Read the model definition and answer for the solid it produces. Units are mm, in the model's axes. Face numbers are marked on the shaded views. Coordinates: 2 decimals unless noted, no trailing zeros. Loops run counter-clockwise (first coordinate to the right, second up) from the corner with the lowest first, then second, coordinate; pieces in that order, holes last. Notation, with made-up numbers: (-35, 2) -> (-1, 2) arc R17 ccw to (-1, 35) -> close; hole circle Ø11 at (65, -11). An arc over 180 degrees is marked (long way). Answer as a JSON object with one key per item and string values. Group by question number.
Q1. Determine the mould class of the marked faces 1, 2, 3 and 4 for opening direction Y: released by +Y, released by -Y, zero draft, split by the parting line, or undercut.
Q2. Straight lines are drawn through the part: line 1 along Y through (x, z) = (0, -3.3) (3 decimals); line 2 along Z through (x, y) = (0, 10.5) (3 decimals); line 3 along Y through (x, z) = (3, -7). For each, find the intervals that lie inside material, in ascending order. Write a range as [from, to].
Q3. The part is cut by section D-D on x = 0.75. Write down the section's boundary in (y, z).
Q4. The part is cut by section B-B on y = 10.25. Write down the section's boundary in (x, z) (3 decimals), and give its area (3 significant figures).
Q5. The part is cut by section A-A on y = 7. Write down the section's boundary in (x, z) (3 decimals).
Q6. Each of these flat-tipped pins is pushed along its axis until it touches: P1, Ø2.5, axis at x = 0, y = 10, coming from the -Z side; P2, Ø6, axis at y = 9.5, z = 12.5, coming from the -X side; P3, Ø4, axis at x = 1.5, z = 11, coming from the -Y side. Where does it stop, or does it pass through?
Q7. The part is cut by section C-C on z = -4. Write down the section's boundary in (x, y) (3 decimals), and give its area (3 significant figures).
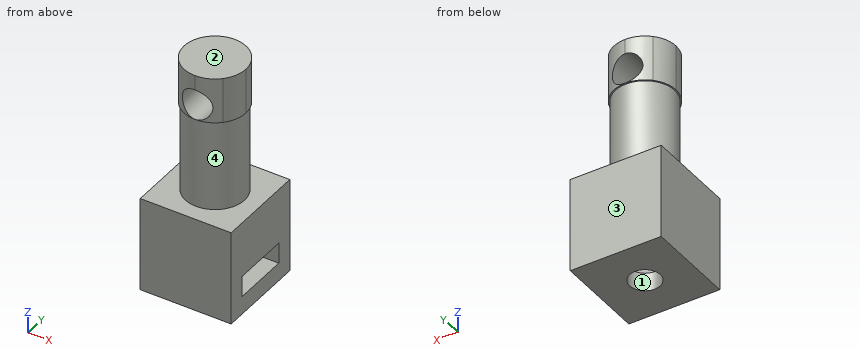
from build123d import *

# Parameters (mm, degrees)
SKETCH1_W               = 10
SKETCH1_H               = 10
BOSS_EXTRUDE1_DEPTH     = 5
CUT_EXTRUDE1_DEPTH      = 9.660254038
CUT_EXTRUDE1_DEPTH_BACK = 9.660254038
SKETCH2_R               = 1.675
SKETCH3_R               = 1.675
CUT_EXTRUDE3_DEPTH      = 2.3
SKETCH4_W               = 10
SKETCH4_H               = 10
BOSS_EXTRUDE2_DEPTH     = 2.7
SKETCH6_W               = 10
SKETCH6_H               = 10
BOSS_EXTRUDE3_DEPTH     = 7
SKETCH9_R               = 2.15
CUT_EXTRUDE12_DEPTH     = 19.468622038
SKETCH10_R              = 1.675
CUT_EXTRUDE13_DEPTH     = 13.003749414
BOSS_EXTRUDE4_DEPTH     = 2.3
SKETCH12_W              = 10
SKETCH12_H              = 10
BOSS_EXTRUDE5_DEPTH     = 2.7
CUT_EXTRUDE14_START     = -2.7
SKETCH13_R              = 1.675
CUT_EXTRUDE14_DEPTH     = 2.7
SKETCH14_R              = 2.15
BOSS_EXTRUDE6_DEPTH     = 0.76
SKETCH16_W              = 10
SKETCH16_H              = 19.7
CUT_EXTRUDE15_DEPTH     = 2.29
BOSS_EXTRUDE7_START     = 1
SKETCH17_W              = 10
SKETCH17_H              = 7.71
SKETCH17_R              = 1.675
BOSS_EXTRUDE7_DEPTH     = 1
SKETCH18_W              = 10
SKETCH18_H              = 7.71
SKETCH18_R              = 1.675
BOSS_EXTRUDE9_DEPTH     = 1
BOSS_EXTRUDE13_DEPTH    = 2.3
SKETCH23_W              = 10
SKETCH23_H              = 10
SKETCH23_R              = 1.675
BOSS_EXTRUDE15_DEPTH    = 2
SKETCH24_W              = 10
SKETCH24_H              = 5.85
CUT_EXTRUDE16_DEPTH     = 25.448519432
SKETCH25_W              = 10
SKETCH25_H              = 10
BOSS_EXTRUDE16_DEPTH    = 6
SKETCH26_W              = 10
SKETCH26_H              = 10
CUT_EXTRUDE17_DEPTH     = 7.71
SKETCH27_W              = 10
SKETCH27_H              = 10
BOSS_EXTRUDE17_DEPTH    = 6.1
SKETCH28_R              = 3.25
BOSS_EXTRUDE18_DEPTH    = 10
SKETCH29_R              = 1.625
CUT_EXTRUDE18_DEPTH     = 2.7
SKETCH33_W              = 6.8
SKETCH33_H              = 6.8
BOSS_EXTRUDE19_DEPTH    = 5
SKETCH36_R              = 1.675
CUT_EXTRUDE22_DEPTH     = 10
CUT_EXTRUDE23_DEPTH     = 10


with BuildPart() as part:
    # Sketch1 → Boss-Extrude1 (new body)
    with BuildSketch(Plane(origin=(0, 0, 0), x_dir=(1, 0, 0), z_dir=(0, 1, 0))):
        Rectangle(SKETCH1_W, SKETCH1_H)
    extrude(amount=BOSS_EXTRUDE1_DEPTH)

    # Sketch2 → Cut-Extrude1 (cut, two sides: drawn at the far end of the back side and taken through both)
    with BuildSketch(Plane(origin=(0, 5, 0), x_dir=(1, 0, 0), z_dir=(0, 1, 0)).offset(-CUT_EXTRUDE1_DEPTH_BACK)):
        with Locations(Location((0, 0, 0), (0, 0, 270))):
            Circle(SKETCH2_R)
    extrude(amount=CUT_EXTRUDE1_DEPTH + CUT_EXTRUDE1_DEPTH_BACK, mode=Mode.SUBTRACT)

    # Sketch3 → Cut-Extrude3 (cut)
    # profile 1 of 2: a face of its own
    with BuildSketch(Plane(origin=(0, 5, 0), x_dir=(1, 0, 0), z_dir=(0, 1, 0))):
        Polygon((-1.56461923, -2.71), (1.56461923, -2.71), (3.129238459, 0), (1.56461923, 2.71), (-1.56461923, 2.71), (-3.129238459, 0), align=None)
        with Locations(Location((0, 0, 0), (0, 0, 270))):
            Circle(SKETCH3_R, mode=Mode.SUBTRACT)
    # profile 2 of 2: a face of its own
    with BuildSketch(Plane(origin=(0, 5, 0), x_dir=(1, 0, 0), z_dir=(0, 1, 0))):
        Polygon((-1.56461923, -2.71), (-3.129238459, 0), (-3.129238459, -5), (3.129238459, -5), (3.129238459, 0), (1.56461923, -2.71), align=None)
    extrude(amount=-CUT_EXTRUDE3_DEPTH, mode=Mode.SUBTRACT)

    # Sketch4 → Boss-Extrude2 (add)
    with BuildSketch(Plane(origin=(0, 5, 0), x_dir=(1, 0, 0), z_dir=(0, 1, 0))):
        Rectangle(SKETCH4_W, SKETCH4_H)
    extrude(amount=BOSS_EXTRUDE2_DEPTH)

    # Sketch6 → Boss-Extrude3 (add)
    with BuildSketch(Plane(origin=(0, 7.7, 0), x_dir=(1, 0, 0), z_dir=(0, 1, 0))):
        Rectangle(SKETCH6_W, SKETCH6_H)
    extrude(amount=BOSS_EXTRUDE3_DEPTH)

    # Sketch9 → Cut-Extrude12 (cut, through all)
    with BuildSketch(Plane(origin=(0, 0, -5), x_dir=(-1, 0, 0), z_dir=(0, 0, -1))):
        with Locations((0, 9.85)):
            Circle(SKETCH9_R)
    extrude(amount=-CUT_EXTRUDE12_DEPTH, mode=Mode.SUBTRACT)

    # Sketch10 → Cut-Extrude13 (cut, through all)
    with BuildSketch(Plane.XZ.offset(-5)):
        with Locations(Location((0, 0, 0), (0, 0, 90))):
            Circle(SKETCH10_R)
    extrude(amount=-CUT_EXTRUDE13_DEPTH, mode=Mode.SUBTRACT)

    # Sketch11 → Boss-Extrude4 (add)
    with BuildSketch(Plane(origin=(0, 14.7, 0), x_dir=(1, 0, 0), z_dir=(0, 1, 0))):
        Polygon((1.56461923, 2.71), (3.129238459, 0), (3.129238459, -5), (5, -5), (5, 5), (-5, 5), (-5, -5), (-3.129238459, -5), (-3.129238459, 0), (-1.56461923, 2.71), align=None)
    extrude(amount=BOSS_EXTRUDE4_DEPTH)

    # Sketch12 → Boss-Extrude5 (add)
    with BuildSketch(Plane(origin=(0, 17, 0), x_dir=(1, 0, 0), z_dir=(0, 1, 0))):
        Rectangle(SKETCH12_W, SKETCH12_H)
    extrude(amount=BOSS_EXTRUDE5_DEPTH)

    # Sketch13 → Cut-Extrude14 (cut)
    with BuildSketch(Plane(origin=(0, 19.7, 0), x_dir=(1, 0, 0), z_dir=(0, 1, 0)).offset(CUT_EXTRUDE14_START)):
        with Locations(Location((0, 0, 0), (0, 0, 270))):
            Circle(SKETCH13_R)
    extrude(amount=CUT_EXTRUDE14_DEPTH, mode=Mode.SUBTRACT)

    # Sketch16 → Cut-Extrude15 (cut)
    with BuildSketch(Plane.XY.offset(5)):
        with Locations((0, 9.85)):
            Rectangle(SKETCH16_W, SKETCH16_H)
    extrude(amount=-CUT_EXTRUDE15_DEPTH, mode=Mode.SUBTRACT)

    # Sketch17 → Boss-Extrude7 (add)
    with BuildSketch(Plane(origin=(0, 0, 0), x_dir=(-1, 0, 0), z_dir=(0, -1, 0)).offset(BOSS_EXTRUDE7_START)):
        with Locations((0, 1.145)):
            Rectangle(SKETCH17_W, SKETCH17_H)
        with Locations(Location((0, 0, 0), (0, 0, 270))):
            Circle(SKETCH17_R, mode=Mode.SUBTRACT)
    extrude(amount=-BOSS_EXTRUDE7_DEPTH)

    # Sketch18 → Boss-Extrude9 (add)
    with BuildSketch(Plane(origin=(0, 19.7, 0), x_dir=(1, 0, 0), z_dir=(0, 1, 0))):
        with Locations((0, 1.145)):
            Rectangle(SKETCH18_W, SKETCH18_H)
        with Locations(Location((0, 0, 0), (0, 0, 270))):
            Circle(SKETCH18_R, mode=Mode.SUBTRACT)
    extrude(amount=BOSS_EXTRUDE9_DEPTH)


with BuildPart() as body_2:
    # Sketch14 → Boss-Extrude6 (new body)
    with BuildSketch(Plane(origin=(0, 0, -5), x_dir=(-1, 0, 0), z_dir=(0, 0, -1))):
        with Locations((0, 9.85)):
            Circle(SKETCH14_R)
    extrude(amount=-BOSS_EXTRUDE6_DEPTH)


    add(part.part)  # Boss-Extrude13 merges part
    # Sketch22 → Boss-Extrude13 (add)
    with BuildSketch(Plane(origin=(0, 0, -5), x_dir=(-1, 0, 0), z_dir=(0, 0, -1))):
        Polygon((-5, 12.979238459), (0, 12.979238459), (2.71, 11.41461923), (2.71, 8.28538077), (0, 6.720761541), (-5, 6.720761541), (-5, 4.85), (5, 4.85), (5, 14.85), (-5, 14.85), align=None)
    extrude(amount=BOSS_EXTRUDE13_DEPTH)

    # Sketch23 → Boss-Extrude15 (add)
    with BuildSketch(Plane(origin=(0, 0, -7.3), x_dir=(-1, 0, 0), z_dir=(0, 0, -1))):
        with Locations((0, 9.85)):
            Rectangle(SKETCH23_W, SKETCH23_H)
        with Locations((0, 9.85)):
            Circle(SKETCH23_R, mode=Mode.SUBTRACT)
    extrude(amount=BOSS_EXTRUDE15_DEPTH)

    # Sketch24 → Cut-Extrude16 (cut, through all)
    with BuildSketch(Plane(origin=(0, 0, -9.3), x_dir=(-1, 0, 0), z_dir=(0, 0, -1))):
        with Locations((0, 17.775)):
            Rectangle(SKETCH24_W, SKETCH24_H)
        with Locations((0, 1.925)):
            Rectangle(SKETCH24_W, SKETCH24_H)
    extrude(amount=-CUT_EXTRUDE16_DEPTH, mode=Mode.SUBTRACT)

    # Sketch25 → Boss-Extrude16 (add)
    with BuildSketch(Plane.XY.offset(2.71)):
        with Locations((0, 9.85)):
            Rectangle(SKETCH25_W, SKETCH25_H)
    extrude(amount=-BOSS_EXTRUDE16_DEPTH)

    # Sketch26 → Cut-Extrude17 (cut)
    with BuildSketch(Plane.XY.offset(2.71)):
        with Locations((0, 9.85)):
            Rectangle(SKETCH26_W, SKETCH26_H)
    extrude(amount=-CUT_EXTRUDE17_DEPTH, mode=Mode.SUBTRACT)

    # Sketch27 → Boss-Extrude17 (add)
    with BuildSketch(Plane.XY.offset(-5)):
        with Locations((0, 9.85)):
            Rectangle(SKETCH27_W, SKETCH27_H)
    extrude(amount=BOSS_EXTRUDE17_DEPTH)

    # Sketch28 → Boss-Extrude18 (add)
    with BuildSketch(Plane.XY.offset(1.1)):
        with Locations((0, 9.85)):
            Circle(SKETCH28_R)
    extrude(amount=BOSS_EXTRUDE18_DEPTH)

    # Sketch29 → Cut-Extrude18 (cut)
    with BuildSketch(Plane(origin=(0, 0, -5), x_dir=(-1, 0, 0), z_dir=(0, 0, -1))):
        with Locations((0, 9.85)):
            Circle(SKETCH29_R)
    extrude(amount=-CUT_EXTRUDE18_DEPTH, mode=Mode.SUBTRACT)

    # Sketch33 → Boss-Extrude19 (add)
    with BuildSketch(Plane.XY.offset(11.1)):
        with Locations((0, 9.85)):
            Rectangle(SKETCH33_W, SKETCH33_H)
    extrude(amount=BOSS_EXTRUDE19_DEPTH)

    # Sketch36 → Cut-Extrude22 (cut)
    with BuildSketch(Plane(origin=(0, 6.45, 0), x_dir=(-1, 0, 0), z_dir=(0, -1, 0))):
        with Locations(Location((0, -12.79, 0), (0, 0, 90))):
            Circle(SKETCH36_R)
    extrude(amount=-CUT_EXTRUDE22_DEPTH, mode=Mode.SUBTRACT)

    # Sketch37 → Cut-Extrude23 (cut)
    with BuildSketch(Plane.XY.offset(16.1)):
        with BuildLine():
            Line((0, 13.25), (-3.4, 13.25))
            Line((-3.4, 13.25), (-2.404163056, 12.254163056))
            ThreePointArc((-2.404163056, 12.254163056), (-1.30112367, 12.991190411), (0, 13.25))
        make_face()
        with BuildLine():
            Line((-2.404163056, 12.254163056), (-3.4, 13.25))
            Line((-3.4, 13.25), (-3.4, 9.85))
            ThreePointArc((-3.4, 9.85), (-3.141190411, 11.15112367), (-2.404163056, 12.254163056))
        make_face()
        with BuildLine():
            ThreePointArc((0, 6.45), (-2.404163056, 7.445836944), (-3.4, 9.85))
            Line((-3.4, 9.85), (-3.4, 6.45))
            Line((-3.4, 6.45), (0, 6.45))
        make_face()
        with BuildLine():
            Line((3.4, 6.45), (2.404163056, 7.445836944))
            ThreePointArc((2.404163056, 7.445836944), (1.30112367, 6.708809589), (0, 6.45))
            Line((0, 6.45), (3.4, 6.45))
        make_face()
        with BuildLine():
            ThreePointArc((3.4, 9.85), (3.141190411, 8.54887633), (2.404163056, 7.445836944))
            Line((2.404163056, 7.445836944), (3.4, 6.45))
            Line((3.4, 6.45), (3.4, 9.85))
        make_face()
        with BuildLine():
            Line((3.4, 13.25), (0, 13.25))
            ThreePointArc((0, 13.25), (2.404163056, 12.254163056), (3.4, 9.85))
            Line((3.4, 9.85), (3.4, 13.25))
        make_face()
    extrude(amount=-CUT_EXTRUDE23_DEPTH, mode=Mode.SUBTRACT)


solid = body_2.part
Final values:
{
 "1": {"face 1": "undercut", "face 2": "zero draft", "face 3": "released by +Y", "face 4": "split by the parting line"},
 "2": {"line 1": "y = [4.85, 8.225], [11.475, 14.85]", "line 2": "z = [-2.3, 11.115], [14.465, 16.1]", "line 3": "y = [4.85, 6.72], [12.98, 14.85]"},
 "3": {"outline": "(4.85, -9.3) -> (8.35, -9.3) -> (8.35, -7.3) -> (6.72, -7.3) -> (6.72, -5) -> (8.41, -5) -> (8.41, -2.3) -> (11.29, -2.3) -> (11.29, -5) -> (12.98, -5) -> (12.98, -7.3) -> (11.35, -7.3) -> (11.35, -9.3) -> (14.85, -9.3) -> (14.85, 1.1) -> (13.01, 1.1) -> (13.01, 11.1) -> (13.17, 11.1) -> (13.17, 11.29) -> (6.53, 11.29) -> (6.53, 11.1) -> (6.69, 11.1) -> (6.69, 1.1) -> (4.85, 1.1) -> close; (6.53, 14.29) -> (13.17, 14.29) -> (13.17, 16.1) -> (6.53, 16.1) -> close"},
 "4": {"outline": "(-5, -9.3) -> (-1.627, -9.3) -> (-1.627, -7.3) -> (-2.71, -7.3) -> (-2.71, -5) -> (-1.575, -5) -> (-1.575, -2.3) -> (1.575, -2.3) -> (1.575, -5) -> (5, -5) -> (5, 1.1) -> (3.225, 1.1) -> (3.225, 11.1) -> (3.376, 11.1) -> (3.376, 16.1) -> (-3.376, 16.1) -> (-3.376, 11.1) -> (-3.225, 11.1) -> (-3.225, 1.1) -> (-5, 1.1) -> close; (1.627, -9.3) -> (5, -9.3) -> (5, -7.3) -> (1.627, -7.3) -> close; hole circle Ø3.35 at (0, 12.79)", "area": "161 mm2"},
 "5": {"outline": "(-5, -9.3) -> (5, -9.3) -> (5, -7.3) -> (-0.484, -7.3) -> (-0.484, -5) -> (5, -5) -> (5, 1.1) -> (1.562, 1.1) -> (1.562, 11.1) -> (1.854, 11.1) -> (1.854, 16.1) -> (-1.854, 16.1) -> (-1.854, 11.1) -> (-1.562, 11.1) -> (-1.562, 1.1) -> (-5, 1.1) -> close; hole circle Ø3.35 at (0, 12.79)"},
 "6": {"P1": "stops at z = -2.3", "P2": "stops at x = -3.4", "P3": "stops at y = 6.45"},
 "7": {"outline": "(-5, 4.85) -> (5, 4.85) -> (5, 14.85) -> (-5, 14.85) -> close; hole circle Ø3.25 at (0, 9.85)", "area": "91.7 mm2"}
}
